from build123d import *

# Parameters (mm, degrees)
PAD_DEPTH       = 16.5
SKETCH001_R     = 6.5
POCKET_DEPTH    = 1.5
SKETCH002_W     = 86
SKETCH002_H     = 2.2
POCKET001_DEPTH = 32
POCKET002_DEPTH = 4
SKETCH004_W     = 4
SKETCH004_H     = 2
SKETCH004_W_2   = 4.5
SKETCH004_H_2   = 3.5
SKETCH004_W_3   = 45.5
POCKET003_DEPTH = 20.5
FILLET_R        = 1


with BuildPart() as part:
    # Sketch → Pad (new body)
    with BuildSketch(Plane.XY):
        with BuildLine():
            Line((-47.5, 33), (-47.5, 3))
            ThreePointArc((-47.5, 3), (-46.62132, 0.87868), (-44.5, 0))
            Line((-44.5, 0), (44.5, 0))
            ThreePointArc((44.5, 0), (46.62132, 0.87868), (47.5, 3))
            Line((47.5, 3), (47.5, 33))
            ThreePointArc((47.5, 33), (46.62132, 35.12132), (44.5, 36))
            Line((44.5, 36), (-44.5, 36))
            ThreePointArc((-44.5, 36), (-46.62132, 35.12132), (-47.5, 33))
        make_face()
    extrude(amount=PAD_DEPTH)

    # Sketch001 (on Face9 of Pad) → Pocket (cut)
    with BuildSketch(Plane(origin=(0, 0, 0), x_dir=(1, 0, 0), z_dir=(0, 0, -1))):
        with Locations((-39.5, -28)):
            Circle(SKETCH001_R)
        with Locations((39.5, -28)):
            Circle(SKETCH001_R)
    extrude(amount=-POCKET_DEPTH, mode=Mode.SUBTRACT)

    # Sketch002 (on Face7 of Pocket) → Pocket001 (cut)
    with BuildSketch(Plane.XZ):
        with Locations((0, 13.6)):
            Rectangle(SKETCH002_W, SKETCH002_H)
    extrude(amount=-POCKET001_DEPTH, mode=Mode.SUBTRACT)

    # Sketch003 (on Face5 of Pocket001) → Pocket002 (cut)
    with BuildSketch(Plane.XY.offset(16.5)):
        with BuildLine():
            Line((-40.5, 0), (40.5, 0))
            ThreePointArc((38, 2.5), (38.732233, 0.732233), (40.5, 0))
            Line((38, 2.5), (38, 31))
            ThreePointArc((38, 31), (37.267767, 32.767767), (35.5, 33.5))
            Line((35.5, 33.5), (-35.5, 33.5))
            ThreePointArc((-35.5, 33.5), (-37.267767, 32.767767), (-38, 31))
            Line((-38, 31), (-38, 2.5))
            ThreePointArc((-40.5, 0), (-38.732233, 0.732233), (-38, 2.5))
        make_face()
    extrude(amount=-POCKET002_DEPTH, mode=Mode.SUBTRACT)

    # Sketch004 (on Face7 of Pocket002) → Pocket003 (cut)
    with BuildSketch(Plane.XZ):
        with Locations((-29.75, 11.5)):
            Rectangle(SKETCH004_W, SKETCH004_H)
        with Locations((29.75, 11.5)):
            Rectangle(SKETCH004_W, SKETCH004_H)
        with Locations((-36.95, 10.75)):
            Rectangle(SKETCH004_W_2, SKETCH004_H_2)
        with Locations((36.95, 10.75)):
            Rectangle(SKETCH004_W_2, SKETCH004_H_2)
        with Locations((0, 11.5)):
            Rectangle(SKETCH004_W_3, SKETCH004_H)
    extrude(amount=-POCKET003_DEPTH, mode=Mode.SUBTRACT)

    # Fillet
    fillet_edges = [part.edges().sort_by_distance(p)[0] for p in [
        (0, 0, 0),
        (0, 36, 16.5),
    ]]
    fillet(fillet_edges, radius=FILLET_R)


solid = part.part
Could you check a few things on this model? Use its own coordinates, in mm. A direction names the side the tool comes from. Coordinates: 2 decimals unless noted, no trailing zeros. Order: outer loops, then holes, each group sorted by start corner. A loop starts at its lowest first (then second) coordinate and runs counter-clockwise, first axis right, second up. Notation, with made-up numbers: (74, 57) -> (111, 57) arc R17 cw to (111, 83) -> close; hole circle Ø6 at (-23, 2.5). An arc over 180 degrees is marked (long way). One line per item, written item: value. Start each with the question number.
1) I'm going to push flat-ended pins straight in: pin 1 (1.3 mm diameter, centred on x = -37, y = 9.5, fed in from +Z); pin 2 (1.5 mm diameter, centred on x = -27, z = 14.5, fed in from -Y); pin 3 (1 mm diameter, centred on x = -30.5, z = 12, fed in from -Y). Where does each tip first touch, or does it pass through?
2) If I drill on L1, parallel to X at y = 28, z = 1.15; L2, parallel to X at y = 4.5, z = 11.75; L3, parallel to Z at x = 40.5, y = 30.5, over which ranges is the centre line in solid material (lowest first)? Write a range as [from, to].
3) We'd pull the mould along X, two halves only. Please class faces 4 (the cylindrical face through (-46.64, 0.9, 8.15)), 5 (the flat face through (-1, 18, 0)), 6 (the flat face through (-37, 20.5, 11)): +X half, -X half, draft (parallel to the pull), parting line (faces both ways), or undercut.
4) Imagine slicing it at C-C on y = 25.5. List the corners of the cut face in (x, z) for me, plus the area to 3 significant figures.
5) Which directions (+Z, -Z, +X, -X, +Y, -Y) give clear straight access to the entire face, cutting with the end or side of a thin tool? Please do faces 1 (the cylindrical face through (-46, 28, 1)), 2 (the flat face through (37, 10, 9)), 3 (the flat face through (31.75, 10, 11)).
6) Imagine slicing it at A-A on z = 13.75. List the corners of the cut face in (x, y) for me.
7) Imagine slicing it at B-B on x = -16. List the corners of the cut face in (y, z) for me, plus the area to 3 significant figures.
Answer list:
1. pin 1: stops at z = 9
1. pin 2: stops at y = 33.5
1. pin 3: stops at y = 20.5
2. L1: x = [-47.5, -46], [-33, 33], [46, 47.5]
2. L2: x = [-47.5, -39.2], [-34.7, -31.75], [-27.75, -22.75], [22.75, 27.75], [31.75, 34.7], [39.2, 47.5]
2. L3: z = [1.5, 12.5], [14.7, 16.5]
3. face 4: -X half
3. face 5: draft
3. face 6: undercut
4. outline: (-47.5, 1) arc R1 ccw to (-46.5, 0) -> (-45.5, 0) -> (-45.5, 1.5) -> (-33.5, 1.5) -> (-33.5, 0) -> (33.5, 0) -> (33.5, 1.5) -> (45.5, 1.5) -> (45.5, 0) -> (46.5, 0) arc R1 ccw to (47.5, 1) -> (47.5, 15.5) arc R1 ccw to (46.5, 16.5) -> (39, 16.5) arc R1 ccw to (38, 15.5) -> (38, 14.7) -> (43, 14.7) -> (43, 12.5) -> (-43, 12.5) -> (-43, 14.7) -> (-38, 14.7) -> (-38, 15.5) arc R1 ccw to (-39, 16.5) -> (-46.5, 16.5) arc R1 ccw to (-47.5, 15.5) -> close
4. area: 1,200 mm2
5. face 1: -Z
5. face 2: -Y
5. face 3: +Z, -Y
6. outline: (-47.5, 3) arc R3 ccw to (-44.5, 0) -> (-43, 0) -> (-43, 32) -> (-37.79, 32) arc R2.5 cw to (-35.5, 33.5) -> (35.5, 33.5) arc R2.5 cw to (37.79, 32) -> (43, 32) -> (43, 0) -> (44.5, 0) arc R3 ccw to (47.5, 3) -> (47.5, 33) arc R3 ccw to (44.5, 36) -> (-44.5, 36) arc R3 ccw to (-47.5, 33) -> close
7. outline: (0, 1) arc R1 ccw to (1, 0) -> (35, 0) arc R1 ccw to (36, 1) -> (36, 15.5) arc R1 ccw to (35, 16.5) -> (34.5, 16.5) arc R1 ccw to (33.5, 15.5) -> (33.5, 12.5) -> (20.5, 12.5) -> (20.5, 10.5) -> (0, 10.5) -> close
7. area: 418 mm2
